```python
from build123d import *

# Parameters (mm, degrees)
F1_W     = 21.59
F1_H     = 2.54
F1_R     = 8.89
F2_DEPTH = 6.35


# Not quite as in the source:
# - a variable given as a bare number and used for a length is read in inches; the dataset says mm whatever the document's units were


with BuildPart() as f2:
    # F1 (on Front) → F2 (new body)
    with BuildSketch(Plane.XZ):
        with BuildLine():
            Line((-50.8, 0), (0, 0))
            Line((0, 0), (50.8, 0))
            Line((50.8, 0), (57.15, -12.7))
            Line((57.15, -12.7), (67.15, -12.7))
            Line((67.15, -12.7), (67.15, 1.825))
            Line((67.15, 1.825), (60.8, 1.825))
            Line((60.8, 1.825), (60.8, 8.175))
            Line((60.8, 8.175), (67.15, 8.175))
            Line((67.15, 8.175), (67.15, 82.55))
            ThreePointArc((67.15, 82.55), (63.4302561211, 91.5302561211), (54.45, 95.25))
            Line((54.45, 95.25), (48.1170043349, 95.25))
            Line((48.1170043349, 95.25), (29.05, 95.25))
            Line((29.05, 95.25), (29.05, 88.9))
            Line((29.05, 88.9), (22.7, 88.9))
            Line((22.7, 88.9), (22.7, 95.25))
            Line((22.7, 95.25), (0, 95.25))
            Line((0, 95.25), (-22.7, 95.25))
            Line((-22.7, 95.25), (-22.7, 88.9))
            Line((-22.7, 88.9), (-29.05, 88.9))
            Line((-29.05, 88.9), (-29.05, 95.25))
            Line((-29.05, 95.25), (-48.1170043349, 95.25))
            Line((-48.1170043349, 95.25), (-54.45, 95.25))
            ThreePointArc((-54.45, 95.25), (-63.4302561211, 91.5302561211), (-67.15, 82.55))
            Line((-67.15, 82.55), (-67.15, 70.6480368972))
            Line((-67.15, 70.6480368972), (-67.15, 8.175))
            Line((-67.15, 8.175), (-60.8, 8.175))
            Line((-60.8, 8.175), (-60.8, 1.825))
            Line((-60.8, 1.825), (-67.15, 1.825))
            Line((-67.15, 1.825), (-67.15, -12.7))
            Line((-67.15, -12.7), (-57.15, -12.7))
            Line((-57.15, -12.7), (-50.8, 0))
        make_face()
        with Locations((53.2934233144, 12.7932670589)):
            Rectangle(F1_W, F1_H, mode=Mode.SUBTRACT)
        with Locations((53.2707386515, 16.3491947024)):
            Rectangle(F1_W, F1_H, mode=Mode.SUBTRACT)
        with Locations((53.2480539886, 19.9051223459)):
            Rectangle(F1_W, F1_H, mode=Mode.SUBTRACT)
        with Locations((53.2253693257, 23.4610499895)):
            Rectangle(F1_W, F1_H, mode=Mode.SUBTRACT)
        with Locations((53.2026846629, 27.016977633)):
            Rectangle(F1_W, F1_H, mode=Mode.SUBTRACT)
        with Locations((53.18, 30.5729052765)):
            Rectangle(F1_W, F1_H, mode=Mode.SUBTRACT)
        Polygon((-54.45, 10), (-54.45, 82.55), (0, 82.55), (39.21, 82.55), (39.21, 10), (0, 10), align=None, mode=Mode.SUBTRACT)
        with Locations((53.18, 47.4004052765)):
            Circle(F1_R, mode=Mode.SUBTRACT)
        with Locations((53.18, 70.2604052765)):
            Circle(F1_R, mode=Mode.SUBTRACT)
    extrude(amount=F2_DEPTH)


solid = f2.part
```
Check sheet for the modelled part. Datum: model origin and axes. Units: mm. A direction names the side the tool comes from. Round coordinates to 2 decimals unless told otherwise and drop trailing zeros. Write each loop counter-clockwise with the first axis right and the second up, starting at its lowest first coordinate (ties: lowest second). Pieces come first, ordered by that corner, then holes. Notation, with made-up numbers: (-25.75, 11) -> (1.25, 11) arc R28 cw to (1.25, 36) -> close; hole circle Ø6 at (25.25, 31.5). An arc over 180 degrees is marked (long way). Put each result on its own line as item: value.
(1) Mould release check, pull along X, two halves, no side actions. Record for faces 1 (the face through (53, -3, 29.303)), 2 (the face through (-67.15, -3, 46)), 3 (the face through (63.53, -3.13, 91.43)), 4 (the face through (64, -3, 1.825)): released by +X, released by -X, zero draft, split by the parting line, or undercut.
Values found:
face 1: undercut
face 2: released by -X
face 3: released by +X
face 4: zero draft
(2) Go/stop test with flat-tipped pins: pin 1 Ø1.9 at (y, z) = (-3, 5) entering from -X; pin 2 Ø1.9 at (x, y) = (-63, -3) entering from +Z; pin 3 Ø3 at (x, y) = (-8, -2.5) entering from -Z. Record where each tip stops, or that it passes through.
Values found:
pin 1: stops at x = -60.8
pin 2: stops at z = 92.72
pin 3: stops at z = 0
(3) Sectioned sample at A-A (x = 6.5). Enter the section's corners in (y, z), plus the area to 3 significant figures.
Values found:
outline: (-6.35, 0) -> (0, 0) -> (0, 10) -> (-6.35, 10) -> close; (-6.35, 82.55) -> (0, 82.55) -> (0, 95.25) -> (-6.35, 95.25) -> close
area: 144 mm^2
(4) Tool access check on faces 5 (the face through (0, -3, 95.25)), 6 (the face through (29.05, -3, 92)), 7 (the face through (-8, -3, 82.55)), 8 (the face through (53.93, -3.13, -6.26)). Record the directions out of +Z, -Z, +X, -X, +Y, -Y that give a thin tool (end or side, any length) a straight path to the whole face; none if there is none.
Values found:
face 5: +Z, +X, -X, +Y, -Y
face 6: +Z, +Y, -Y
face 7: +Y, -Y
face 8: -Z, +Y, -Y
(5) Material ranges on line 1 (X direction, y = -1.75, z = 26); line 2 (X direction, y = -3, z = 20.5); line 3 (Z direction, x = 17.5, y = -5.25), recorded low to high.
Values found:
line 1: x = -67.15 to -54.45, 39.21 to 42.41, 64 to 67.15
line 2: x = -67.15 to -54.45, 39.21 to 42.45, 64.04 to 67.15
line 3: z = 0 to 10, 82.55 to 95.25
(6) Sectioned sample at C-C (y = -4.5). Count the separate pieces of the cut face and the enclosed holes in it, plus the area to 3 significant figures.
Values found:
separate pieces: 1
enclosed holes: 9
area: 5,280 mm^2
(7) Sectioned sample at B-B (z = 43). Enter the section's corners in (x, y), plus the area to 3 significant figures.
Values found:
outline: (-67.15, -6.35) -> (-54.45, -6.35) -> (-54.45, 0) -> (-67.15, 0) -> close; (39.21, -6.35) -> (45.46, -6.35) -> (45.46, 0) -> (39.21, 0) -> close; (60.9, -6.35) -> (67.15, -6.35) -> (67.15, 0) -> (60.9, 0) -> close
area: 160 mm^2
